Part model, mm, in its own coordinate system. Face numbers are marked on the shaded views. A direction names the side the tool comes from. Give positions to 0.01 mm unless a question says otherwise; leave off trailing zeros. Order: outer loops, then holes, each group sorted by start corner. A loop starts at its lowest first (then second) coordinate and runs counter-clockwise, first axis right, second up.
1. Which spindle directions (+Z, -Z, +X, -X, +Y, -Y) get a long thin tool onto all of the face, cutting with end or side? Do the marked faces 1, 2 and 3. Say none if no direction does.
2. Slice it at A-A on z = 0. List the corners of the cut face in (x, y).
3. Slice it at C-C on y = 2.75. List the corners of the cut face in (x, z).
4. Probe line 1 (Y direction, x = 1, z = 1.75); line 2 (Y direction, x = 0, z = 1.5); line 3 (X direction, y = 1.75, z = 2). List the from-to ranges inside material, lowest first.
5. Drop flat-ended pins along their axis: pin 1 Ø4 at (x, y) = (-0.5, 4) entering from -Z; pin 2 Ø0.6 at (x, z) = (0, 0.5) entering from -Y; pin 3 Ø5 at (x, y) = (0.5, 4) entering from +Z. Give the stop position or say it passes through.
6. Slice it at B-B on x = 0. List the corners of the cut face in (y, z), and give its area (3 significant figures).
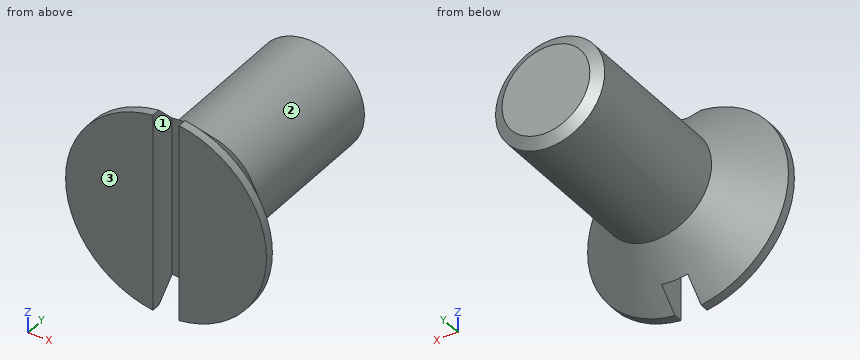
from build123d import *

# Parameters (mm, degrees)
SKETCH001_W  = 9.2
SKETCH001_H  = 1.2
POCKET_DEPTH = 1.3


with BuildPart() as part:
    # Sketch → Revolution (revolve)
    with BuildSketch(Plane.YZ):
        Polygon((0, 0), (0, 4.6), (0.4, 4.6), (2.5, 2.5), (9.717098, 2.5), (10, 2.01), (10, 0), align=None)
    revolve(axis=Axis((0, 0, 0), (0, 1, 0)))

    # Sketch001 → Pocket (cut)
    with BuildSketch(Plane(origin=(0, 0, 0), x_dir=(0, 0, -1), z_dir=(0, -1, 0))):
        Rectangle(SKETCH001_W, SKETCH001_H)
    extrude(amount=-POCKET_DEPTH, mode=Mode.SUBTRACT)


solid = part.part
Data:
1. face 1: +Z, -Z, -Y
1. face 2: +Y
1. face 3: +Z, -Z, +X, -X, -Y
2. outline: (-4.6, 0) - (-0.6, 0) - (-0.6, 1.3) - (0.6, 1.3) - (0.6, 0) - (4.6, 0) - (4.6, 0.4) - (2.5, 2.5) - (2.5, 9.72) - (2.01, 10) - (-2.01, 10) - (-2.5, 9.72) - (-2.5, 2.5) - (-4.6, 0.4) - close
3. outline: circle Ø5 at (0, 0)
4. line 1: y = 0 to 10
4. line 2: y = 1.3 to 10
4. line 3: x = -2.56 to 2.56
5. pin 1: stops at z = -2.97
5. pin 2: stops at y = 1.3
5. pin 3: stops at z = 3.48
6. outline: (1.3, -3.7) - (2.5, -2.5) - (9.72, -2.5) - (10, -2.01) - (10, 2.01) - (9.72, 2.5) - (2.5, 2.5) - (1.3, 3.7) - close
6. area: 44.8 mm2
